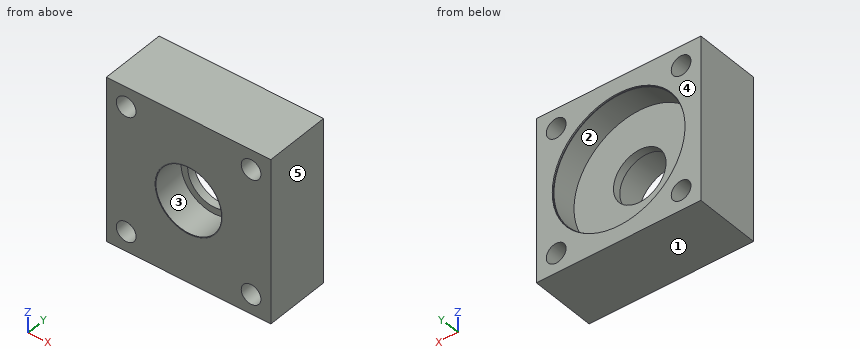
Autodesk Inventor part; units mm, degrees
ref_plane "YZ Plane" through (0, 0, 0) normal (1, 0, 0) x (0, 1, 0)
ref_plane "XZ Plane" through (0, 0, 0) normal (0, 1, 0) x (-1, 0, 0)
ref_plane "XY Plane" through (0, 0, 0) normal (0, 0, 1) x (1, 0, 0)
sketch "Sketch1" plane through (0, 0, 0) normal (0, 1, 0) x (-1, 0, 0)
  circle A0 centre (0, 0) radius 5.08
  line L0 (-15.875, 15.875) -> (15.875, 15.875)
  line L1 (15.875, 15.875) -> (15.875, -15.875)
  line L2 (15.875, -15.875) -> (-15.875, -15.875)
  line L3 (-15.875, -15.875) -> (-15.875, 15.875)
  line L4 (-15.875, 15.875) -> (15.875, -15.875) construction
  line L5 (15.875, 15.875) -> (-15.875, -15.875) construction
  dimension "d0" = 10.16
  dimension "d1" = 31.75
  dimension "d2" = 31.75
extrude "Extrusion1" add sketch "Sketch1" along normal blind 12.7
sketch "Sketch2" plane through (0, 12.7, 0) normal (0, 1, 0) x (1, 0, 0)
  circle A0 centre (0, 0) radius 12.7
  dimension "d5" = 25.4
extrude "Extrusion2" cut sketch "Sketch2" against normal blind 5.08
sketch "Sketch3" plane through (0, 12.7, 0) normal (0, 1, 0) x (1, 0, 0)
  line L0 (-12.065, 12.065) -> (12.065, 12.065) construction
  line L1 (12.065, 12.065) -> (12.065, -12.065) construction
  line L2 (12.065, -12.065) -> (-12.065, -12.065) construction
  line L3 (-12.065, -12.065) -> (-12.065, 12.065) construction
  line L4 (-12.065, 12.065) -> (12.065, -12.065) construction
  line L5 (12.065, 12.065) -> (-12.065, -12.065) construction
  line L6 (15.875, -15.875) -> (15.875, 15.875)
  line L7 (-15.875, -15.875) -> (15.875, -15.875)
  point P0 (0, 0)
  dimension "d8" = 3.81
  dimension "d9" = 3.81
hole "Hole1" at (12.065, 12.7, 12.065) at (-12.065, 12.7, 12.065) at (-12.065, 12.7, -12.065) at (12.065, 12.7, -12.065) direction (0, -1, 0) diameter 3.81 end through all
sketch "Sketch4" plane through (0, 12.7, 0) normal (0, 1, 0) x (1, 0, 0)
  circle A0 centre (0, 0) radius 12.827
  dimension "d17" = 25.654
extrude "Extrusion3" cut sketch "Sketch4" against normal blind 0.254
sketch "Sketch5" plane through (0, 0, 0) normal (0, -1, 0) x (1, 0, 0)
  circle A0 centre (0, 0) radius 6.477
  dimension "d20" = 12.954
extrude "Extrusion4" cut sketch "Sketch5" against normal blind 0.0508
sketch "Sketch6" plane through (0, 0, 0) normal (0, -1, 0) x (1, 0, 0)
  circle A0 centre (0, 0) radius 6.35
  dimension "d23" = 12.7
extrude "Extrusion5" cut sketch "Sketch6" against normal blind 6.096
properties part number "silverSolderJoint" material "Copper"
Design review of the part built by this model. Coordinates are the model's own, in mm. Face numbers are marked on the shaded views. A direction names the side the tool comes from. Coordinates: 2 decimals unless noted, no trailing zeros. Order: outer loops, then holes, each group sorted by start corner. A loop starts at its lowest first (then second) coordinate and runs counter-clockwise, first axis right, second up. Notation, with made-up numbers: (-24, 5) -> (23, 5) arc R9 ccw to (23, 11) -> close; hole circle Ø7 at (15, 57). An arc over 180 degrees is marked (long way). Use one line per item in the form item = value. Start each with the question number.
(1) Add section C-C on z = 11. Give the number of separate pieces and of enclosed holes in the cut face, plus the area to 3 significant figures.
(2) Add section A-A on x = 0. State the section outline as (y, z) points (3 decimals).
(3) For the marked faces 1 and 2, list the 3-axis set-ups (+Z, -Z, +X, -X, +Y, -Y) from which the entire face can be reached by the end or side of a thin tool; tool diameter is ignored.
(4) Add section D-D on y = 12. State the section outline as (x, z) points (3 decimals).
(5) The part is to be moulded in two halves that separate along X. For the marked faces 3, 4 and 5, say which applies: +X half, -X half, draft (parallel to the pull), parting line (faces both ways), or undercut.
(6) Insertion check: pin 1 (4 mm diameter, centred on x = -1, z = 0.5, fed in from -Y). The pin has a flat end and moves straight along its axis. Give the tip position at first contact, or say it passes through.
(7) For probe 1 along X at (y, z) = (4, 12) (3 decimals); probe 2 along X at (y, z) = (6, 13) (3 decimals); probe 3 along Z at (x, y) = (0, 9.5) (3 decimals), list the stretches that pass through material, from the lowest coordinate up.
(8) Add section B-B on z = 0. State the section outline as (x, y) points (3 decimals), plus the area to 3 significant figures.
Answer block:
q1.separate_pieces = 3
q1.enclosed_holes = 0
q1.area = 258 mm²
q2.outline = (0, -15.875) -> (12.7, -15.875) -> (12.7, -12.827) -> (12.446, -12.827) -> (12.446, -12.7) -> (7.62, -12.7) -> (7.62, -5.08) -> (6.096, -5.08) -> (6.096, -6.35) -> (0.051, -6.35) -> (0.051, -6.477) -> (0, -6.477) -> close; (0, 6.477) -> (0.051, 6.477) -> (0.051, 6.35) -> (6.096, 6.35) -> (6.096, 5.08) -> (7.62, 5.08) -> (7.62, 12.7) -> (12.446, 12.7) -> (12.446, 12.827) -> (12.7, 12.827) -> (12.7, 15.875) -> (0, 15.875) -> close
q3.face_1 = -Z, +X, -X, +Y, -Y
q3.face_2 = +Y
q4.outline = (-15.875, -15.875) -> (15.875, -15.875) -> (15.875, 15.875) -> (-15.875, 15.875) -> close; hole circle Ø3.81 at (-12.065, -12.065); hole circle Ø3.81 at (-12.065, 12.065); hole circle Ø25.4 at (0, 0); hole circle Ø3.81 at (12.065, -12.065); hole circle Ø3.81 at (12.065, 12.065)
q5.face_3 = undercut
q5.face_4 = draft
q5.face_5 = +X half
q6.pin_1 = through
q7.probe_1 = -15.875 to -13.969, -10.161 to 10.161, 13.969 to 15.875
q7.probe_2 = -15.875 to -13.725, -10.405 to 10.405, 13.725 to 15.875
q7.probe_3 = -15.875 to -12.7, 12.7 to 15.875
q8.outline = (-15.875, 0) -> (-6.477, 0) -> (-6.477, 0.051) -> (-6.35, 0.051) -> (-6.35, 6.096) -> (-5.08, 6.096) -> (-5.08, 7.62) -> (-12.7, 7.62) -> (-12.7, 12.446) -> (-12.827, 12.446) -> (-12.827, 12.7) -> (-15.875, 12.7) -> close; (5.08, 6.096) -> (6.35, 6.096) -> (6.35, 0.051) -> (6.477, 0.051) -> (6.477, 0) -> (15.875, 0) -> (15.875, 12.7) -> (12.827, 12.7) -> (12.827, 12.446) -> (12.7, 12.446) -> (12.7, 7.62) -> (5.08, 7.62) -> close
q8.area = 181 mm²
